from build123d import *

# Parameters (mm, degrees)
SKETCH1_R           = 30
BOSS_EXTRUDE1_DEPTH = 30
SKETCH2_W           = 60
SKETCH2_H           = 90
BOSS_EXTRUDE2_DEPTH = 15
SKETCH3_R           = 8
BOSS_EXTRUDE3_DEPTH = 15


with BuildPart() as part:
    # Sketch1 → Boss-Extrude1 (new body)
    with BuildSketch(Plane.XY):
        Circle(SKETCH1_R)
        with BuildLine():
            Line((-4, -14.456832295), (-4, -17.956832295))
            Line((-4, -17.956832295), (4, -17.956832295))
            Line((4, -17.956832295), (4, -14.456832295))
            ThreePointArc((4, -14.456832295), (0, 15), (-4, -14.456832295))
        make_face(mode=Mode.SUBTRACT)
    extrude(amount=-BOSS_EXTRUDE1_DEPTH)

    # Sketch2 → Boss-Extrude2 (add)
    with BuildSketch(Plane(origin=(0, 0, -30), x_dir=(-1, 0, 0), z_dir=(0, 0, -1))):
        Rectangle(SKETCH2_W, SKETCH2_H)
    extrude(amount=BOSS_EXTRUDE2_DEPTH)

    # Sketch3 → Boss-Extrude3 (add)
    with BuildSketch(Plane(origin=(0, 45, 0), x_dir=(1, 0, 0), z_dir=(0, 1, 0))):
        with BuildLine():
            Line((22.03289839, 71.599347585), (30, 45))
            Line((30, 45), (30, 30))
            Line((30, 30), (-30, 30))
            Line((-30, 30), (-30, 45))
            Line((-30, 45), (-22.03289839, 71.599347585))
            ThreePointArc((-22.03289839, 71.599347585), (0, 88), (22.03289839, 71.599347585))
        make_face()
        with Locations(Location((0, 65, 0), (0, 0, 180))):
            Circle(SKETCH3_R, mode=Mode.SUBTRACT)
    boss_extrude3 = extrude(amount=-BOSS_EXTRUDE3_DEPTH)

    # Mirror1: Boss-Extrude3 across plane
    add(boss_extrude3.mirror(Plane.ZX))


solid = part.part
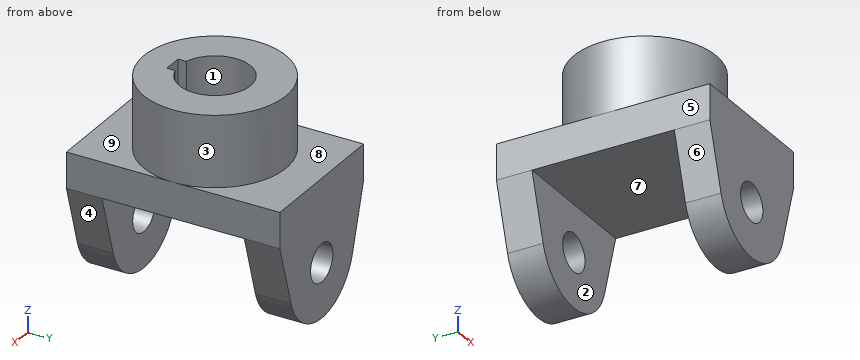
Verification items for the finished model (mm, model axes). Face numbers are marked on the shaded views. A direction names the side the tool comes from. Give positions to 0.01 mm unless a question says otherwise; leave off trailing zeros. Loops run counter-clockwise (first coordinate to the right, second up) from the corner with the lowest first, then second, coordinate; pieces in that order, holes last.
1) Sectioned sample at B-B, the plane z = -55.5. Enter the section's corners in (x, y), then the cut area to 3 significant figures.
2) Sectioned sample at D-D, the plane z = -65. Enter the section's corners in (x, y), then the cut area to 3 significant figures.
3) Depth check by flat-ended pin: pin 1 Ø9.5 at (x, z) = (0, -65) entering from +Y; pin 2 Ø9 at (x, z) = (1, -11) entering from +Y; pin 3 Ø3 at (y, z) = (-16.5, -20) entering from +X; pin 4 Ø3 at (x, z) = (-12.5, -14.5) entering from -Y. Enter the tip coordinate at first touch or a pass-through.
4) Set-up check for the marked faces 5, 6, 7, 8 and 9: record each of +Z, -Z, +X, -X, +Y, -Y from which the full face is reachable in a straight line by a thin tool's end or side.
5) Sectioned sample at A-A, the plane x = 0. Enter the section's corners in (y, z), then the cut area to 3 significant figures.
6) Draft check along Y on the marked faces 1, 2, 3 and 4. Enter one of: pulls with the +Y half, pulls with the -Y half, needs draft (parallel to the pull), parting line crosses it, or undercut.
7) Sectioned sample at C-C, the plane y = 34.5. Enter the section's corners in (x, z), then the cut area to 3 significant figures.
8) Thickness scan on line 1 along Y through (x, z) = (20, -55); line 2 along Z through (x, y) = (0, 40.5); line 3 along Z through (x, y) = (-5, -28). Record the ranges inside material, lowest first.
Answers:
1. outline: (-26.86, -45) - (26.86, -45) - (26.86, -30) - (-26.86, -30) - close; (-26.86, 30) - (26.86, 30) - (26.86, 45) - (-26.86, 45) - close
1. area: 1,610 mm2
2. outline: (-24.01, -45) - (-8, -45) - (-8, -30) - (-24.01, -30) - close; (-24.01, 30) - (-8, 30) - (-8, 45) - (-24.01, 45) - close; (8, -45) - (24.01, -45) - (24.01, -30) - (8, -30) - close; (8, 30) - (24.01, 30) - (24.01, 45) - (8, 45) - close
2. area: 961 mm2
3. pin 1: passes through
3. pin 2: stops at y = 30
3. pin 3: stops at x = 25.98
3. pin 4: stops at y = -27.91
4. face 5: +Z, -Z, -X, +Y, -Y
4. face 6: -Z, -X, +Y, -Y
4. face 7: -Z, +X, -X
4. face 8: +Z, +Y
4. face 9: +Z, -Y
5. outline: (-45, -88) - (-30, -88) - (-30, -73) - (-45, -73) - close; (-45, -57) - (-30, -57) - (-30, -45) - (30, -45) - (30, -57) - (45, -57) - (45, -30) - (30, -30) - (30, 0) - (15, 0) - (15, -30) - (-17.96, -30) - (-17.96, 0) - (-30, 0) - (-30, -30) - (-45, -30) - close; (30, -88) - (45, -88) - (45, -73) - (30, -73) - close
5. area: 2,970 mm2
6. face 1: undercut
6. face 2: undercut
6. face 3: parting line crosses it
6. face 4: needs draft
7. outline: (-30, -45) - (-22.03, -71.6) arc R23 ccw to (22.03, -71.6) - (30, -45) - (30, -30) - (-30, -30) - close; hole circle Ø16 at (0, -65)
7. area: 2,610 mm2
8. line 1: y = -45 to -30, 30 to 45
8. line 2: z = -88 to -73, -57 to -30
8. line 3: z = -45 to 0
